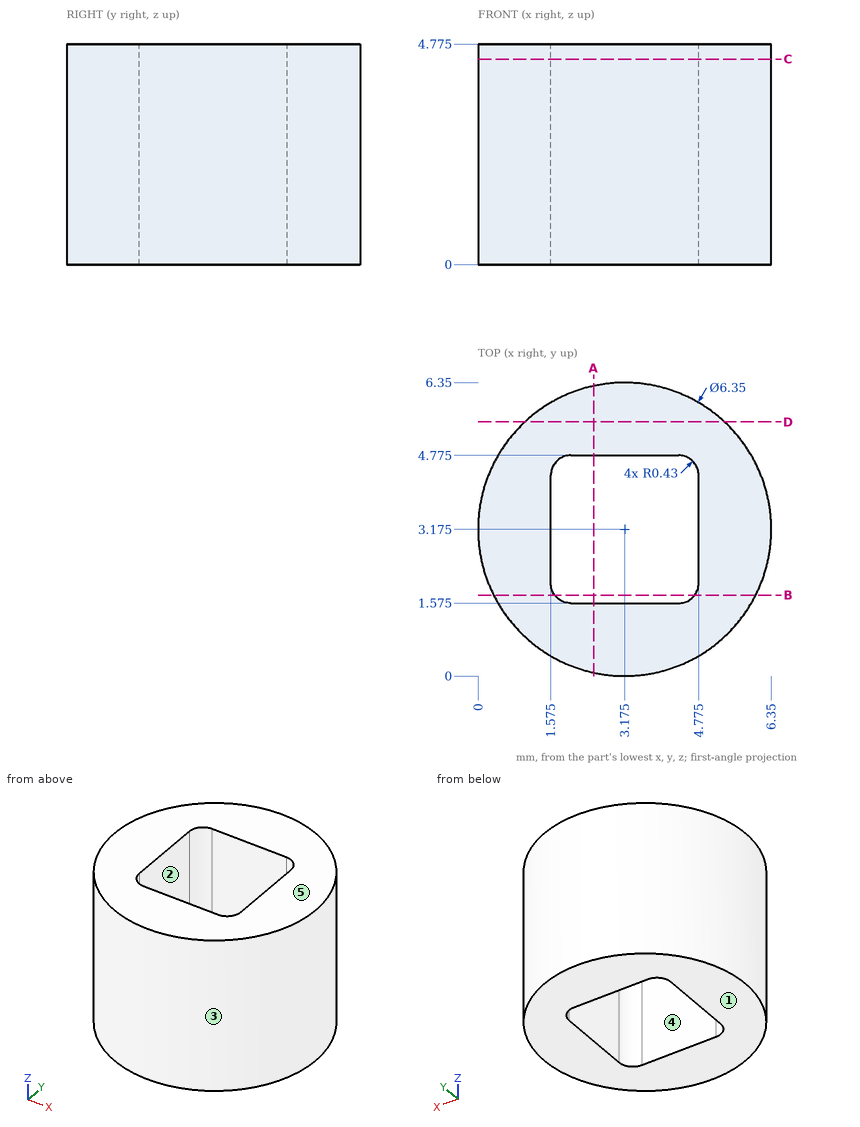
Input: dimensioned drawing with shaded views. Units: mm. Origin: part minimum x, y, z. A direction names the side the tool comes from. Round coordinates to 2 decimals unless told otherwise and drop trailing zeros. Loops run counter-clockwise (first coordinate to the right, second up) from the corner with the lowest first, then second, coordinate; pieces in that order, holes last. Notation, with made-up numbers: (24, 19) -> (43, 19) arc R25 cw to (43, 37) -> close; hole circle Ø9 at (-16.75, 46.5). An arc over 180 degrees is marked (long way). Answer as a JSON object with one key per item and string values. Group by question number.
Q1. Section query A-A (x = 2.5). Output: boundary loops of the cut face in (y, z) (1 decimal).
Q2. Mould query, pull axis X, two halves, no side actions, for the marked faces 3, 4 and 5. Classes: pulls with the +X half, pulls with the -X half, needs draft (parallel to the pull), parting line crosses it, or undercut.
Q3. Section query D-D (y = 5.5). Output: boundary loops of the cut face in (x, z) (1 decimal).
Q4. Contact query for flat-ended pins moving along their axis: P1, Ø2, axis at x = 1, z = 3, coming from the +Y side (1 decimal); P2, Ø1.5, axis at x = 1, z = 3.5, coming from the +Y side; P3, Ø0.7, axis at y = 2.5, z = 3, coming from the -X side. Output: stop coordinate, or through.
Q5. Section query C-C (z = 4.45). Output: boundary loops of the cut face in (x, y) (3 decimals).
Q6. Ray query, line 1 (X direction, y = 3.25, z = 0.75) (1 decimal); line 2 (Y direction, x = 2, z = 2.7) (1 decimal); line 3 (X direction, y = 4.5, z = 0.25). Return the intervals inside material, ascending. Write a range as from..to.
Q7. Access query for the marked faces 1 and 2. Directions: +Z, -Z, +X, -X, +Y, -Y. A direction counts if a zero-diameter tool reaches every point of the face in a straight line with its end or side. Return the directions, or none.
Q8. Section query B-B (y = 1.75). Output: boundary loops of the cut face in (x, z) (1 decimal), plus the area to 3 significant figures.
Completed:
{
 "1": {"outline": "(0.1, 0) -> (1.6, 0) -> (1.6, 4.8) -> (0.1, 4.8) -> close; (4.8, 0) -> (6.3, 0) -> (6.3, 4.8) -> (4.8, 4.8) -> close"},
 "2": {"face 3": "parting line crosses it", "face 4": "undercut", "face 5": "needs draft"},
 "3": {"outline": "(1, 0) -> (5.3, 0) -> (5.3, 4.8) -> (1, 4.8) -> close"},
 "4": {"P1": "y = 6.1", "P2": "y = 6.01", "P3": "x = 0.02"},
 "5": {"outline": "circle Ø6.35 at (3.175, 3.175); hole (1.575, 2.005) arc R0.43 ccw to (2.005, 1.575) -> (4.345, 1.575) arc R0.43 ccw to (4.775, 2.005) -> (4.775, 4.345) arc R0.43 ccw to (4.345, 4.775) -> (2.005, 4.775) arc R0.43 ccw to (1.575, 4.345) -> close"},
 "6": {"line 1": "0..1.6, 4.8..6.3", "line 2": "0.2..1.6, 4.8..6.1", "line 3": "0.29..1.6, 4.75..6.06"},
 "7": {"face 1": "-Z, +X, -X, +Y, -Y", "face 2": "+Z, -Z"},
 "8": {"outline": "(0.3, 0) -> (1.7, 0) -> (1.7, 4.8) -> (0.3, 4.8) -> close; (4.7, 0) -> (6, 0) -> (6, 4.8) -> (4.7, 4.8) -> close", "area": "12.6 mm²"}
}
